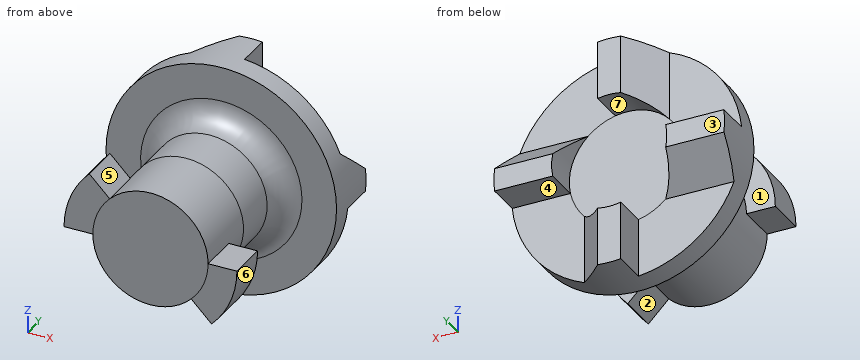
```python
from build123d import *
from build123d.topology import SkipClean

# Parameters (mm, degrees)
SKETCH1_R               = 5
BOSS_EXTRUDE1_DEPTH     = 6
BOSS_EXTRUDE5_START     = 6
SKETCH11_R              = 5
BOSS_EXTRUDE5_DEPTH     = 6
SKETCH2_R               = 10
BOSS_EXTRUDE2_DEPTH     = 2
BOSS_EXTRUDE3_DEPTH     = 3
BOSS_EXTRUDE4_REACH     = 26.92
CIRPATTERN1_COUNT       = 4
CUT_EXTRUDE3_DEPTH      = 20.8997487421324
CUT_EXTRUDE3_DEPTH_BACK = 20.8997487421324
SKETCH10_R              = 13.301263658979888
FILLET1_R               = 2
CUT_EXTRUDE4_START      = -3
SKETCH12_R              = 5
CUT_EXTRUDE4_DEPTH      = 3
BOSS_EXTRUDE6_DEPTH     = 3.5


with BuildPart() as part:
    # Sketch1 → Boss-Extrude1 (new body)
    with BuildSketch(Plane(origin=(0, 0, 0), x_dir=(1, 0, 0), z_dir=(0, 1, 0))):
        with Locations(Location((0, 0, 0), (0, 0, 270))):
            Circle(SKETCH1_R)
    extrude(amount=BOSS_EXTRUDE1_DEPTH)

    # Sketch11 → Boss-Extrude5 (add)
    with BuildSketch(Plane.XZ.offset(BOSS_EXTRUDE5_START)):
        with Locations(Location((0, 0, 0), (0, 0, 270))):
            Circle(SKETCH11_R)
    extrude(amount=-BOSS_EXTRUDE5_DEPTH)

    # Sketch2 → Boss-Extrude2 (add)
    with BuildSketch(Plane(origin=(0, 6, 0), x_dir=(1, 0, 0), z_dir=(0, 1, 0))):
        with Locations(Location((0, 0, 0), (0, 0, 270))):
            Circle(SKETCH2_R)
    extrude(amount=BOSS_EXTRUDE2_DEPTH)

    # Sketch4 → Boss-Extrude3 (add)
    with BuildSketch(Plane(origin=(0, 8, 0), x_dir=(1, 0, 0), z_dir=(0, 1, 0))):
        with BuildLine():
            Line((1, 9.999999999999998), (-1, 9.999999999999998))
            Line((-1, 9.999999999999998), (-1, 4.898979485566357))
            ThreePointArc((-1, 4.898979485566357), (-3.5355339059327378, 3.5355339059327386), (-4.898979485566357, 1))
            Line((-4.898979485566357, 1), (-10, 1.0000000000000004))
            Line((-10, 1.0000000000000004), (-10, -1))
            Line((-10, -1), (-4.898979485566357, -1))
            ThreePointArc((-4.898979485566357, -1), (-3.5355339059327378, -3.5355339059327386), (-1, -4.898979485566356))
            Line((-1, -4.898979485566356), (-1.0000000000000002, -10.000000000000002))
            Line((-1.0000000000000002, -10.000000000000002), (1.0000000000000002, -10))
            Line((1.0000000000000002, -10), (1, -4.898979485566356))
            ThreePointArc((1, -4.898979485566356), (3.5355339059327378, -3.5355339059327373), (4.898979485566357, -1))
            Line((4.898979485566357, -1), (10, -1))
            Line((10, -1), (10, 1))
            Line((10, 1), (4.898979485566357, 1))
            ThreePointArc((4.898979485566357, 1), (3.5355339059327378, 3.5355339059327386), (1, 4.898979485566357))
            Line((1, 4.898979485566357), (1, 9.999999999999998))
        make_face()
    extrude(amount=BOSS_EXTRUDE3_DEPTH)

    # Sketch9 → Boss-Extrude4 (add, up to next)
    with BuildSketch(Plane(origin=(0, 0, -9.999999999999998), x_dir=(-1, 0, 0), z_dir=(0, 0, -1)), mode=Mode.PRIVATE) as boss_extrude4_sk1:
        Polygon((-1, 11), (-3.7012121328935463, 8), (-1.000000000000001, 8), align=None)
    boss_extrude4_tool1 = extrude(boss_extrude4_sk1.sketch, amount=-BOSS_EXTRUDE4_REACH, mode=Mode.PRIVATE) - part.part
    boss_extrude4 = boss_extrude4_tool1.solids().sort_by_distance((1.900404, 9, -10))[0]
    add(boss_extrude4)

    # CirPattern1: Boss-Extrude4 ×4 about axis
    cirpattern1_axis = Axis((0, 0, 1.47e-15), (0, 1, 0))
    for i in range(1, CIRPATTERN1_COUNT):
        add(boss_extrude4.rotate(cirpattern1_axis, i * 360 / CIRPATTERN1_COUNT))

    # Sketch10 → Cut-Extrude3 (cut, two sides: drawn at the far end of the back side and taken through both)
    with BuildSketch(Plane(origin=(0, 8, 0), x_dir=(1, 0, 0), z_dir=(0, 1, 0)).offset(-CUT_EXTRUDE3_DEPTH_BACK)):
        Circle(SKETCH10_R)
        with BuildLine():
            ThreePointArc((9.9498743710662, 0.9999999999999999), (9.987460731103328, 0.5006277505981886), (10, 0))
            ThreePointArc((10, -2.45e-15), (-8.276838808655619, -5.611946127283498), (3.7012121328935477, 9.289834699676932))
            ThreePointArc((3.701212132893546, 9.28983469967693), (7.985510661293986, 6.019270676615241), (9.9498743710662, 1))
        make_face(mode=Mode.SUBTRACT)
    extrude(amount=CUT_EXTRUDE3_DEPTH + CUT_EXTRUDE3_DEPTH_BACK, mode=Mode.SUBTRACT)

    # Fillet1
    fillet1_edges = [part.edges().sort_by_distance(p)[0] for p in [
        (1.53e-15, 6, -5),
    ]]
    fillet(fillet1_edges, radius=FILLET1_R)

    # Sketch12 → Cut-Extrude4 (cut)
    with SkipClean():  # the faces are left unmerged after this step: merging them gives an invalid solid
        with BuildSketch(Plane(origin=(0, 11, 0), x_dir=(1, 0, 0), z_dir=(0, 1, 0)).offset(CUT_EXTRUDE4_START)):
            with Locations(Location((0, 0, 0), (0, 0, 90))):
                Circle(SKETCH12_R)
        extrude(amount=CUT_EXTRUDE4_DEPTH, mode=Mode.SUBTRACT)

    # Sketch14 → Boss-Extrude6 (add)
    with SkipClean():  # the faces are left unmerged after this step: merging them gives an invalid solid
        with BuildSketch(Plane.XZ.offset(6)):
            with BuildLine():
                ThreePointArc((-5, 6.1e-16), (-4.619397662556429, 1.9134171618254616), (-3.535533905932718, 3.535533905932757))
                Line((-3.535533905932719, 3.5355339059327564), (-5.303300858899078, 5.303300858899133))
                ThreePointArc((-5.303300858899077, 5.303300858899135), (-6.929096493834643, 2.8701257427381925), (-7.5, 9.2e-16))
                Line((-7.5, -2.4e-16), (-5, 0))
            make_face()
            with BuildLine():
                Line((7.5, -2.4e-16), (5, 0))
                ThreePointArc((5, -1.22e-15), (4.619397662556436, -1.9134171618254436), (3.535533905932746, -3.535533905932729))
                Line((3.535533905932746, -3.5355339059327293), (5.303300858899117, -5.303300858899095))
                ThreePointArc((5.3033008588991155, -5.303300858899099), (6.9290964938346535, -2.8701257427381655), (7.5, -1.84e-15))
            make_face()
        extrude(amount=-BOSS_EXTRUDE6_DEPTH)


solid = part.part
```
Model file for the job. Use its own axes, mm. Face numbers are marked on the shaded views. A direction names the side the tool comes from. Coordinates: 2 decimals unless noted, no trailing zeros. Loops run counter-clockwise (first coordinate to the right, second up) from the corner with the lowest first, then second, coordinate; pieces in that order, holes last. Notation, with made-up numbers: M 29,65 L 37,65 A24 ccw 37,84 Z; hole C 80.25,81 d9. An arc over 180 degrees is marked long. Use CSV: the item, a comma, the result in double quotes. Start each with the question number.
1. Tool access for the marked faces 4, 5, 6 and 7: list every direction of +Z, -Z, +X, -X, +Y, -Y with a clear straight run to the whole face (end or side of a thin tool).
2. Band-saw the part on A-A, the plane y = -4. List the corners of the cut face in (x, z), then the cut area to 3 significant figures.
3. Band-saw the part on C-C, the plane y = 7. List the corners of the cut face in (x, z).
4. Flat gauge pins, fed straight in: pin 1 (1.5 mm diameter, centred on x = 1, y = 1.5, fed in from +Z); pin 2 (5 mm diameter, centred on x = -6.5, z = 6, fed in from +Y); pin 3 (3 mm diameter, centred on x = 8, y = -1, fed in from +Z); pin 4 (5 mm diameter, centred on y = 6.5, z = 3.5, fed in from -X). Where does each tip first touch, or does it go through?
5. Probe probe 1 along Y at (x, z) = (3, 1.75); probe 2 along X at (y, z) = (6.75, -0.25); probe 3 along Y at (x, z) = (5.75, -2). List the from-to ranges inside material, lowest first. Write a range as [from, to].
6. Band-saw the part on B-B, the plane z = -7.75. List the corners of the cut face in (x, y), then the cut area to 3 significant figures.
7. Two-plate mould, pull along Y, no slides. Class the marked faces 1, 2 and 3: pulls with the +Y half, pulls with the -Y half, needs draft (parallel to the pull), parting line crosses it, or undercut.
Entries:
1,face 4,"-Z, +X, +Y"
1,face 5,"+Z, -Y"
1,face 6,"-Z, +X, -Y"
1,face 7,"+Y"
2,outline,"M -7.5,0 L -5,0 A5 ccw 3.54,-3.54 L 5.3,-5.3 A7.5 ccw 7.5,0 L 5,0 A5 ccw -3.54,3.54 L -5.3,5.3 A7.5 ccw Z"
2,area,"103 mm2"
3,outline,"C 0,0 d20"
4,pin 1,"stops at z = 4.99"
4,pin 2,"stops at y = 8"
4,pin 3,"passes through"
4,pin 4,"stops at x = -9.95"
5,probe 1,"y = [-6, 8]"
5,probe 2,"x = [-10, 10]"
5,probe 3,"y = [-6, -2.5], [5.78, 8]"
6,outline,"M -6.32,6 L 6.32,6 L 6.32,8 L 3.7,8 L 1,11 L -1,11 L -1,8 L -6.32,8 Z"
6,area,"35.3 mm2"
7,face 1,"undercut"
7,face 2,"needs draft"
7,face 3,"pulls with the +Y half"
